For this review, take the finished solid that the model builds, in its own axes (mm). A direction names the side the tool comes from. Give positions to 0.01 mm unless a question says otherwise; leave off trailing zeros. Loops run counter-clockwise (first coordinate to the right, second up) from the corner with the lowest first, then second, coordinate; pieces in that order, holes last. Notation, with made-up numbers: (16, 34.25) - (59, 34.25) arc R19 cw to (59, 62.25) - close; hole circle Ø2 at (-14.75, -22.5). An arc over 180 degrees is marked (long way). Put each result on its own line as item: value.
Autodesk Inventor part; units mm, degrees
ref_plane "YZ Plane" through (0, 0, 0) normal (1, 0, 0) x (0, 1, 0)
ref_plane "XZ Plane" through (0, 0, 0) normal (0, 1, 0) x (-1, 0, 0)
ref_plane "XY Plane" through (0, 0, 0) normal (0, 0, 1) x (1, 0, 0)
sketch "Sketch1" plane through (0, 0, 0) normal (0, 0, 1) x (1, 0, 0)
  line L0 (0, 0) -> (38.1, 0)
  line L1 (38.1, 0) -> (38.1, 38.1)
  line L2 (38.1, 38.1) -> (0, 38.1)
  line L3 (0, 38.1) -> (0, 0)
  line L4 (3.175, 34.925) -> (34.925, 34.925)
  line L5 (34.925, 34.925) -> (34.925, 3.175)
  line L6 (34.925, 3.175) -> (3.175, 3.175)
  line L7 (3.175, 3.175) -> (3.175, 34.925)
  dimension "d0" = 38.1
  dimension "d1" = 38.1
  dimension "d2" = 3.175
extrude "Extrusion1" add sketch "Sketch1" along normal blind 177.8
sketch "Sketch2" plane through (0, 38.1, 0) normal (0, 1, 0) x (1, 0, 0)
  line L0 (12.5095, -87.63) -> (25.5905, -87.63)
  line L1 (30.353, -82.8675) -> (30.353, -16.1925)
  line L2 (25.5905, -11.43) -> (12.5095, -11.43)
  line L3 (7.747, -16.1925) -> (7.747, -82.8675)
  line L4 (38.1, 0) -> (0, 0)
  arc A0 (7.747, -82.8675) -> (12.5095, -87.63) centre (12.5095, -82.8675) ccw
  arc A1 (25.5905, -87.63) -> (30.353, -82.8675) centre (25.5905, -82.8675) ccw
  arc A2 (30.353, -16.1925) -> (25.5905, -11.43) centre (25.5905, -16.1925) ccw
  arc A3 (12.5095, -11.43) -> (7.747, -16.1925) centre (12.5095, -16.1925) ccw
  point P0 (30.353, -11.43)
  point P1 (30.353, -87.63)
  point P2 (7.747, -11.43)
  point P3 (19.05, -11.43)
  point P4 (19.05, 0)
  dimension "d5" = 22.606
  dimension "d6" = 76.2
  dimension "d7" = 11.43
  dimension "d8" = 4.7625
extrude "Extrusion2" cut sketch "Sketch2" against normal blind 3.175
sketch "Sketch3" plane through (0, 38.1, 0) normal (0, 1, 0) x (1, 0, 0)
  circle A0 centre (7.112, -10.795) radius 1.289
  line L0 (0, 0) -> (0, -177.8)
  line L1 (12.5095, -11.43) -> (25.5905, -11.43)
  line L2 (7.747, -82.8675) -> (7.747, -16.1925)
  circle A1 centre (30.988, -10.795) radius 1.289
  circle A2 centre (7.112, -88.265) radius 1.289
  circle A3 centre (30.988, -88.265) radius 1.289
  circle A4 centre (5.461, -21.1137) radius 1.2891
  circle A5 centre (32.639, -21.1137) radius 1.2891
  circle A6 centre (5.461, -30.7975) radius 1.2891
  circle A7 centre (32.639, -30.7975) radius 1.2891
  circle A8 centre (5.461, -40.4812) radius 1.2891
  circle A9 centre (32.639, -40.4812) radius 1.2891
  circle A10 centre (5.461, -50.165) radius 1.2891
  circle A11 centre (32.639, -50.165) radius 1.2891
  circle A12 centre (5.461, -59.8487) radius 1.2891
  circle A13 centre (32.639, -59.8487) radius 1.2891
  circle A14 centre (5.461, -69.5325) radius 1.2891
  circle A15 centre (32.639, -69.5325) radius 1.2891
  circle A16 centre (5.461, -79.2162) radius 1.2891
  circle A17 centre (32.639, -79.2162) radius 1.2891
  circle A18 centre (15.7048, -9.144) radius 1.2891
  circle A19 centre (23.6626, -9.144) radius 1.2891
  circle A20 centre (15.7048, -89.916) radius 1.2891
  circle A21 centre (23.6626, -89.916) radius 1.2891
  dimension "d11" = 2.5781
  dimension "d14" = 0.635
  dimension "d15" = 0.635
  dimension "d18" = 23.876
  dimension "d21" = 77.47
  dimension "d24" = 2.5781
  dimension "d25" = 2.286
  dimension "d26" = 9.6837
  dimension "d29" = 27.178
  dimension "d32" = 9.6837
  dimension "d35" = 2.5781
  dimension "d36" = 7.9578
  dimension "d37" = 2.286
  dimension "d40" = 7.9578
  dimension "d43" = 80.772
extrude "Extrusion3" cut sketch "Sketch3" against normal blind 3.175
sketch "Sketch4" plane through (0, 0, 0) normal (0, -1, 0) x (1, 0, 0)
  circle A0 centre (19.05, 82.55) radius 1.2891
  line L0 (0, 0) -> (38.1, 0)
  line L1 (38.1, 0) -> (38.1, 177.8)
  circle A1 centre (19.05, 95.25) radius 1.2891
  point P0 (19.05, 0)
  dimension "d48" = 2.5781
  dimension "d49" = 82.55
  dimension "d52" = 12.7
extrude "Extrusion4" cut sketch "Sketch4" against normal blind 3.175
sketch "Sketch5" plane through (0, 0, 0) normal (0, -1, 0) x (1, 0, 0)
  circle A0 centre (19.05, 114.3) radius 2.3813
  line L0 (0, 0) -> (38.1, 0)
  point P0 (19.05, 0)
  dimension "d59" = 4.7625
  dimension "d60" = 114.3
extrude "Extrusion5" cut sketch "Sketch5" against normal blind 3.175
sketch "Sketch6" plane through (0, 38.1, 0) normal (0, 1, 0) x (1, 0, 0)
  circle A0 centre (9.525, -161.925) radius 4.7625
  line L0 (38.1, -177.8) -> (0, -177.8)
  line L1 (0, 0) -> (0, -177.8)
  circle A1 centre (23.8125, -168.275) radius 4.7625
  line L2 (38.1, 0) -> (38.1, -177.8)
  dimension "d63" = 15.875
  dimension "d64" = 9.525
  dimension "d65" = 9.525
  dimension "d66" = 9.525
  dimension "d67" = 14.2875
  dimension "d68" = 9.525
extrude "Extrusion6" cut sketch "Sketch6" against normal blind 3.175
properties part number "Hull_Alu" material "Aluminum 6061"
1) Take a section at B-B on z = 114.3. State the section outline as (x, y) points (3 decimals).
Geometry check:
outline: (0, 0) - (16.669, 0) - (16.669, 3.175) - (3.175, 3.175) - (3.175, 34.925) - (34.925, 34.925) - (34.925, 3.175) - (21.431, 3.175) - (21.431, 0) - (38.1, 0) - (38.1, 38.1) - (0, 38.1) - close
2) Insertion check: pin 1 Ø1.5 at (x, z) = (32.64, 59.85) entering from +Y (3 decimals). The pin has a flat end and moves straight along its axis. Give the tip position at first contact, or say it passes through.
Geometry check:
pin 1: stops at y = 3.175
3) Take a section at A-A on y = 13.5. State the section outline as (x, z) points (3 decimals), and give its area (3 significant figures).
Geometry check:
outline: (0, 0) - (3.175, 0) - (3.175, 177.8) - (0, 177.8) - close; (34.925, 0) - (38.1, 0) - (38.1, 177.8) - (34.925, 177.8) - close
area: 1,130 mm²
4) Draft analysis for pull direction Y (two halves, no side actions). For faces 1 (the face through (18.534, 1.565, 111.975)), 2 (the face through (19, 38.1, 107)), 3 (the face through (19, 3.175, 88)), state which applies: pulls with the +Y half, pulls with the -Y half, needs draft (parallel to the pull), parting line crosses it, or undercut.
Geometry check:
face 1: needs draft
face 2: pulls with the +Y half
face 3: undercut
5) For faces 4 (the face through (7.747, 37, 49)), 5 (the face through (38.1, 19, 88)), 6 (the face through (3.175, 19, 88)), list the 3-axis set-ups (+Z, -Z, +X, -X, +Y, -Y) from which the entire face can be reached by the end or side of a thin tool; tool diameter is ignored.
Geometry check:
face 4: +Y
face 5: +Z, -Z, +X, +Y, -Y
face 6: +Z, -Z
6) Wall thickness on line 1 (X direction, y = 2.3, z = 82.55); line 2 (Y direction, x = 25, z = 92.5) (3 decimals): over which ranges is each line inside the solid? List them lowest first.
Geometry check:
line 1: x = 0 to 17.76, 20.34 to 38.1
line 2: y = 0 to 3.175, 34.925 to 38.1
